Geometry: final body of the model. Coordinates: model frame, mm. A direction names the side the tool comes from. Give positions to 0.01 mm unless a question says otherwise; leave off trailing zeros. Write each loop counter-clockwise with the first axis right and the second up, starting at its lowest first coordinate (ties: lowest second). Pieces come first, ordered by that corner, then holes. Notation, with made-up numbers: M 47.25,-22 L 73.25,-22 A20 ccw 73.25,-4 Z; hole C 9,-9.75 d8. An arc over 180 degrees is marked long. Use a Markdown table: item, result. Add a question column.
(1) Cut plane A-A (z = -0.25). Output: boundary loops of the cut face in (x, y), plus the area to 3 significant figures.
(2) Draft query along Z for faces 1 (the flat face through (118, 169, 1.588)), 2 (the flat face through (52.2, 229.7, 1.588)), 3 (the flat face through (131.6, 188.5, -4.318)), 4 (the cylindrical face through (159.083, 337.544, 3.723)). Return one class per face: released by +Z, released by -Z, zero draft, split by the parting line, or undercut.
(3) Pin query (flat end, axial travel): pin 1 Ø1 at (y, z) = (128.5, 0) entering from -X; pin 2 Ø1 at (y, z) = (256, 3) entering from +X. Return the tip coordinate at first contact, or that it passes through.
(4) Material intervals for L1, parallel to X at y = 334.5, z = 1.5; L2, parallel to Y at x = 128.5, z = 1.25; L3, parallel to X at y = 263.5, z = -2, sorted ascending.
(5) Reachability of faces 5 (the cylindrical face through (157.5, 340.96, 3.71)), 6 (the flat face through (37.03, 190.22, 3.72)), 7 (the cylindrical face through (13.349, 61.967, -3.706)), 8 (the cylindrical face through (13.6, 62.4, 0)), 9 (the flat face through (107.522, 157.057, 3.723)) from +Z, -Z, +X, -X, +Y, -Y: full face, straight path, thin tool, end or side. Return the list, or none.
Autodesk Inventor part; units mm, degrees
ref_plane "Work Plane2" through (20.602935, 75.239361, 0) normal (-1, 0, 0) x (0, 0, 1)
ref_plane "Work Plane3" through (130.265709, 285.46929, 0) normal (-0.3453892, -0.9384595, 0) x (0, 0, 1)
ref_plane "Section Plane" through (33.368035, 65.144213, 0) normal (0.6203041, 0.7843614, 0) x (0, 0, 1)
ref_plane "Work Plane2" through (20.602935, 75.239361, 0) normal (-1, 0, 0) x (0, 0, 1)
ref_plane "Work Plane3" through (130.265709, 285.46929, 0) normal (-0.3453892, -0.9384595, 0) x (0, 0, 1)
sketch "Path" plane through (0, 0, 0) normal (0, 0, 1) x (1, 0, 0)
  arc A0 (5.019556, 79.931703) -> (33.368035, 65.144213) centre (20.602935, 75.239361) ccw
  arc A1 (177.849583, 247.838078) -> (72.176269, 302.960718) centre (130.265709, 285.46929) ccw
  line L0 (177.849583, 247.838078) -> (33.368035, 65.144213)
  line L1 (5.019556, 79.931703) -> (72.176269, 302.960718)
  dimension "d31" = 5.9944
ref_plane "Section Plane" through (33.368035, 65.144213, 0) normal (0.6203041, 0.7843614, 0) x (0, 0, 1)
sketch "Section Sketch" plane through (33.368035, 65.144213, 0) normal (0.6203041, 0.7843614, 0) x (0, 0, 1)
  line L0 (-4.318, -1.14935) -> (4.318, -1.14935)
  line L1 (4.318, -1.14935) -> (4.318, 1.14935)
  line L2 (4.318, 1.14935) -> (-4.318, 1.14935)
  line L3 (-4.318, 1.14935) -> (-4.318, -1.14935)
  line L4 (-1.5875, -1.651) -> (1.5875, -1.651)
  line L5 (1.5875, -1.651) -> (1.5875, 1.651)
  line L6 (1.5875, 1.651) -> (-1.5875, 1.651)
  line L7 (-1.5875, 1.651) -> (-1.5875, -1.651)
  line L8 (-1.5875, 0) -> (1.5875, 0) construction
  line L9 (-3.1115, -2.9972) -> (-1.5875, -2.9972)
  line L10 (-1.5875, -2.9972) -> (-1.5875, 2.9972)
  line L11 (-1.5875, 2.9972) -> (-3.1115, 2.9972)
  line L12 (-3.1115, 2.9972) -> (-3.1115, -2.9972)
  line L13 (1.5875, -2.9972) -> (3.1115, -2.9972)
  line L14 (3.1115, -2.9972) -> (3.1115, 2.9972)
  line L15 (3.1115, 2.9972) -> (1.5875, 2.9972)
  line L16 (1.5875, 2.9972) -> (1.5875, -2.9972)
  line L17 (-4.318, 0) -> (4.318, 0) construction
  point P0 (0, 0)
  point P1 (0, 0)
  dimension "d21" = 2.2987
  dimension "d22" = 3.302
  dimension "d23" = 3.175
  dimension "d24" = 1.524
  dimension "d31" = 5.9944
  dimension "d32" = 8.636
sweep "Solid" add profiles "Section Sketch" path "Path"
pattern_of_one "Strand Pattern"
equation "\"d21\" = da_d2"
equation "\"d22\" = da_d1"
equation "\"d23\" = da_b1"
equation "\"d24\" = da_t1 + da_t2"
equation "\"d30\" = da_pt"
equation "\"da_p\" = 6.35"
equation "\"da_b1\" = 3.175"
equation "\"da_h2\" = 5.9944"
equation "\"da_h3\" = 5.207"
equation "\"da_d1\" = 3.302"
equation "\"da_d2\" = 2.2987"
equation "\"da_pt\" = 6.4008"
equation "\"da_b\" = 8.636"
equation "\"da_t1\" = 0.762"
equation "\"da_t2\" = 0.762"
properties part number "Roller Chain"
Answer list:
| question | item | result |
|---|---|---|
| 1 | outline | M 3.44,80.41 A17.93 ccw 34.66,64.12 L 179.14,246.81 A62.32 ccw long 70.6,303.44 Z; hole M 6.6,79.46 A14.62 ccw 32.07,66.17 L 176.55,248.86 A59.01 ccw long 73.76,302.48 Z |
| 1 | area | 2,390 mm² |
| 2 | face 1 | undercut |
| 2 | face 2 | undercut |
| 2 | face 3 | released by -Z |
| 2 | face 4 | zero draft |
| 3 | pin 1 | x = 17.77 |
| 3 | pin 2 | x = 186.96 |
| 4 | L1 | 91.8 to 97.42, 163.11 to 168.73 |
| 4 | L2 | 182.77 to 188.1, 344.46 to 347.76 |
| 4 | L3 | 57.16 to 63.42, 183.59 to 190.02 |
| 5 | face 5 | +Z |
| 5 | face 6 | +Z, -X, +Y |
| 5 | face 7 | -Z |
| 5 | face 8 | none |
| 5 | face 9 | +Z, +X, -Y |
